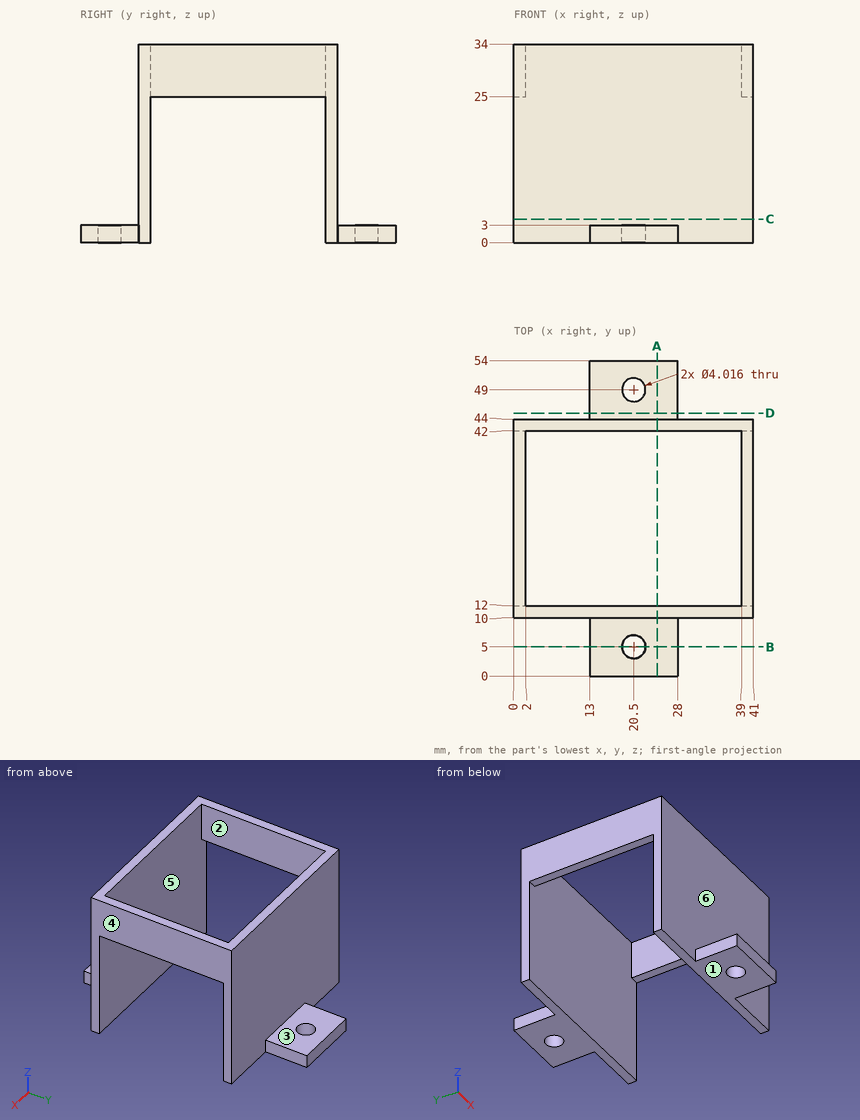
Study the drawing (mm; zero at the part's minimum x, y, z) and answer. A direction names the side the tool comes from. Round coordinates to 2 decimals unless told otherwise and drop trailing zeros. Write each loop counter-clockwise with the first axis right and the second up, starting at its lowest first coordinate (ties: lowest second). Pieces come first, ordered by that corner, then holes.
1) A cutting plane is placed at D-D (y = 45). Give the vertices of the cut face in (x, z), plus the area to 3 significant figures.
2) A tool of negligible diameter and unlimited length cuts with its end or side. For the marked faces 1, 2 and 3, from which of +Z, -Z, +X, -X, +Y, -Y can it reach the whole face along a straight path? Write none if from no direction.
3) A cutting plane is placed at C-C (z = 4). Give the vertices of the cut face in (x, y).
4) Straight lines are drawn through the part: line 1 (Y direction, x = 20.5, z = 2); line 2 (Y direction, x = 12, z = 23.5); line 3 (Y direction, x = 20, z = 2) (1 decimal). For each, find the intervals that lie inside material, in ascending order.
5) A cutting plane is placed at B-B (y = 5). Give the vertices of the cut face in (x, z).
6) The mould has two halves that part along X. Classify the marked faces 4, 5 and 6: pulls with the +X half, pulls with the -X half, needs draft (parallel to the pull), parting line crosses it, or undercut.
7) Given pin 1 Ø5 at (x, y) = (18, 6) entering from +Z; pin 2 Ø17 at (x, z) = (22, 15) entering from +Y; pin 3 Ø8 at (x, z) = (7.5, 25) entering from -Y; pin 4 Ø3 at (x, y) = (20.5, 49) entering from -Z, each flat-ended and moving along its own axis, determine where each tip first touches the part or whether it passes through.
8) A cutting plane is placed at A-A (x = 24.5). Give the vertices of the cut face in (y, z), plus the area to 3 significant figures.
Completed:
1. outline: (13, 0) - (28, 0) - (28, 3) - (13, 3) - close
1. area: 45.0 mm2
2. face 1: -Z, +X, -X, +Y, -Y
2. face 2: +Z, -Z
2. face 3: +Z, +X, -X, +Y
3. outline: (0, 10) - (41, 10) - (41, 12) - (0, 12) - close; (0, 42) - (41, 42) - (41, 44) - (0, 44) - close
4. line 1: y = 0 to 2.99, 7.01 to 12, 42 to 46.99, 51.01 to 54
4. line 2: y = 10 to 12, 42 to 44
4. line 3: y = 0 to 3.1, 6.9 to 12, 42 to 47.1, 50.9 to 54
5. outline: (13, 0) - (18.49, 0) - (18.49, 3) - (13, 3) - close; (22.51, 0) - (28, 0) - (28, 3) - (22.51, 3) - close
6. face 4: pulls with the +X half
6. face 5: undercut
6. face 6: needs draft
7. pin 1: stops at z = 3
7. pin 2: stops at y = 44
7. pin 3: stops at y = 10
7. pin 4: passes through
8. outline: (0, 0) - (12, 0) - (12, 34) - (10, 34) - (10, 3) - (0, 3) - close; (42, 0) - (54, 0) - (54, 3) - (44, 3) - (44, 34) - (42, 34) - close
8. area: 196 mm2
